Autodesk Inventor part; units mm, degrees
ref_plane "YZ Plane" through (0, 0, 0) normal (1, 0, 0) x (0, 1, 0)
ref_plane "XZ Plane" through (0, 0, 0) normal (0, 1, 0) x (-1, 0, 0)
ref_plane "XY Plane" through (0, 0, 0) normal (0, 0, 1) x (1, 0, 0)
sketch "Sketch1" plane through (0, 0, 0) normal (0, 0, 1) x (1, 0, 0)
  circle A0 centre (0, 0) radius 6
  dimension "d0" = 12
extrude "Extrusion1" add sketch "Sketch1" along normal mid plane 67.38
sketch "Sketch2" plane through (0, 0, 33.69) normal (0, 0, 1) x (1, 0, 0)
  circle A0 centre (0, 0) radius 6
hole "Hole1" at (0, 0, 33.69) direction (0, 0, -1) diameter 4.9784 depth 12.7 tip angle 118
mirror "Mirror1" about plane through (0, 0, 0) normal (0, 0, 1) of "Hole1"
properties part number "Dead Axle" material "Steel"
Check sheet for the modelled part. Datum: model origin and axes. Units: mm. A direction names the side the tool comes from. Give positions to 0.01 mm unless a question says otherwise; leave off trailing zeros. Order: outer loops, then holes, each group sorted by start corner. A loop starts at its lowest first (then second) coordinate and runs counter-clockwise, first axis right, second up. Notation, with made-up numbers: M -12,17.25 L 28,17.25 A26 cw 28,48.25 Z; hole C 60,-35.5 d1. An arc over 180 degrees is marked long. Answer in a Markdown table with one row per item.
1) Release check for a two-part mould opening along Y. For faces 4 (the conical face through (0.422, 0.094, -19.754)), 5 (the cylindrical face through (-6, 0, 0)), 6 (the flat face through (3, 0, 33.69)) record: +Y half, -Y half, draft (parallel to the pull), parting line (faces both ways), or undercut.
Filled sheet:
| item | result |
|---|---|
| face 4 | undercut |
| face 5 | parting line |
| face 6 | draft |
2) Cross-section at B-B, the plane z = -17. Enter the section's corners in (x, y).
Filled sheet:
| item | result |
|---|---|
| outline | C 0,0 d12 |
3) Gauge pin test, flat ends, axial feed: P1, Ø6, axis at x = 1, z = 21, coming from the +Y side; P2, Ø4, axis at x = 4, z = 14.5, coming from the +Y side. Record the tip position at first contact, or that the pin passes through.
Filled sheet:
| item | result |
|---|---|
| P1 | stops at y = 6 |
| P2 | stops at y = 5.66 |
4) Cross-section at A-A, the plane z = -26. Enter the section's corners in (x, y).
Filled sheet:
| item | result |
|---|---|
| outline | C 0,0 d12; hole C 0,0 d4.98 |
5) Access from +Z, -Z, +X, -X, +Y, -Y to the whole of each face (thin tool, end or side, straight path). Record for faces 1 (the cylindrical face through (-0.748, -2.374, 27.251)), 2 (the flat face through (3, 0, -33.69)), 3 (the cylindrical face through (0.748, -2.374, -27.251)).
Filled sheet:
| item | result |
|---|---|
| face 1 | +Z |
| face 2 | -Z, +X, -X, +Y, -Y |
| face 3 | -Z |
6) Cross-section at D-D, the plane y = 5.25. Enter the section's corners in (x, z).
Filled sheet:
| item | result |
|---|---|
| outline | M -2.9,-33.69 L 2.9,-33.69 L 2.9,33.69 L -2.9,33.69 Z |
7) Cross-section at C-C, the plane x = 4. Enter the section's corners in (y, z), plus the area to 3 significant figures.
Filled sheet:
| item | result |
|---|---|
| outline | M -4.47,-33.69 L 4.47,-33.69 L 4.47,33.69 L -4.47,33.69 Z |
| area | 603 mm2 |
8) Thickness scan on L1, parallel to Y at x = 0, z = 24; L2, parallel to Y at x = 1.5, z = 27; L3, parallel to X at y = 0.5, z = -27.5. Record the ranges inside material, lowest first. Write a range as [from, to].
Filled sheet:
| item | result |
|---|---|
| L1 | y = [-6, -2.49], [2.49, 6] |
| L2 | y = [-5.81, -1.99], [1.99, 5.81] |
| L3 | x = [-5.98, -2.44], [2.44, 5.98] |
